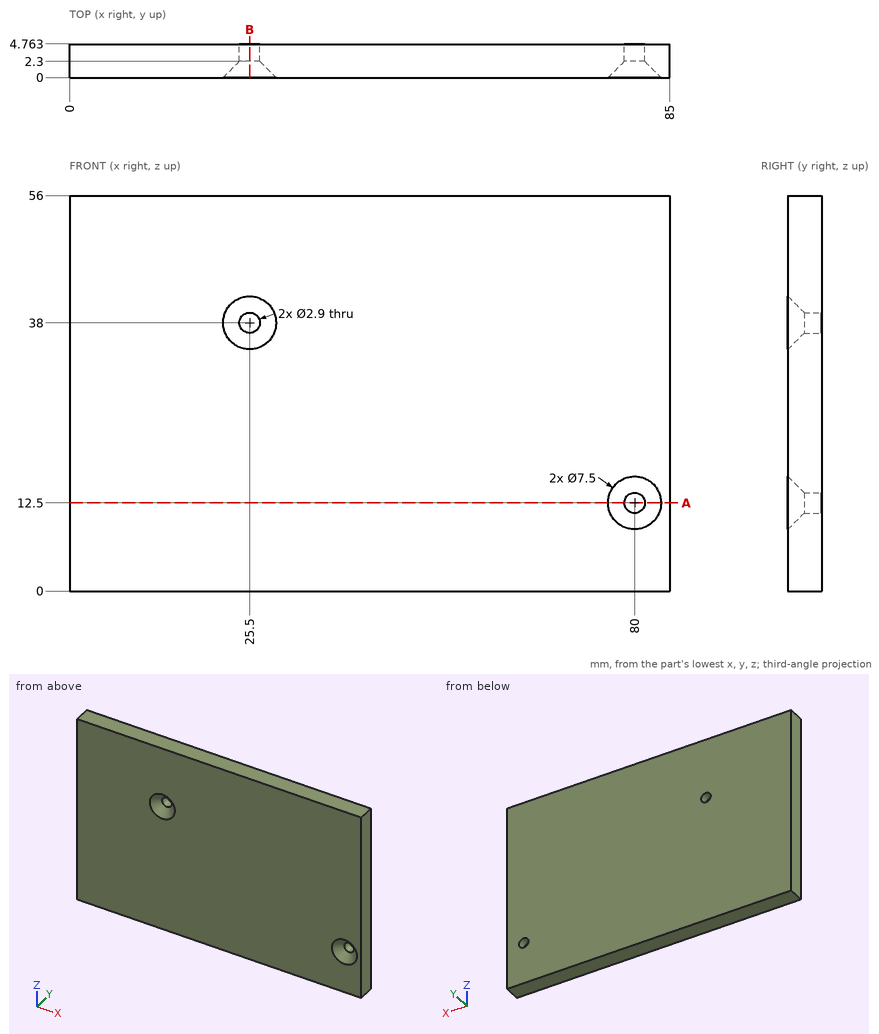
Part print with two shaded views. Sizes in mm from the minimum x, y, z corner. Coordinates: 2 decimals unless noted, no trailing zeros. Write each loop counter-clockwise with the first axis right and the second up, starting at its lowest first coordinate (ties: lowest second). Pieces come first, ordered by that corner, then holes.
(1) Drill centre lines: line 1 (Z direction, x = 25.5, y = 2.95); line 2 (X direction, y = 3.45, z = 38); line 3 (X direction, y = 4.35, z = 12.5). Where is each one in solid material? Low to high.
(2) Cut at A-A on z = 12.5. List the corners of the cut face in (x, y).
(3) Cut at B-B on x = 25.5. List the corners of the cut face in (y, z).
Working result:
1. line 1: z = 0 to 36.55, 39.45 to 56
1. line 2: x = 0 to 24.05, 26.95 to 85
1. line 3: x = 0 to 78.55, 81.45 to 85
2. outline: (0, 0) - (76.25, 0) - (78.55, 2.3) - (78.55, 4.76) - (0, 4.76) - close; (81.45, 2.3) - (83.75, 0) - (85, 0) - (85, 4.76) - (81.45, 4.76) - close
3. outline: (0, 0) - (4.76, 0) - (4.76, 36.55) - (2.3, 36.55) - (0, 34.25) - close; (0, 41.75) - (2.3, 39.45) - (4.76, 39.45) - (4.76, 56) - (0, 56) - close
